Can you work these out from the model? Positions are in its coordinate system, mm. Face numbers are marked on the shaded views. A direction names the side the tool comes from. Give positions to 0.01 mm unless a question says otherwise; leave off trailing zeros. Write each loop counter-clockwise with the first axis right and the second up, starting at its lowest first coordinate (ties: lowest second). Pieces come first, ordered by that corner, then holes.
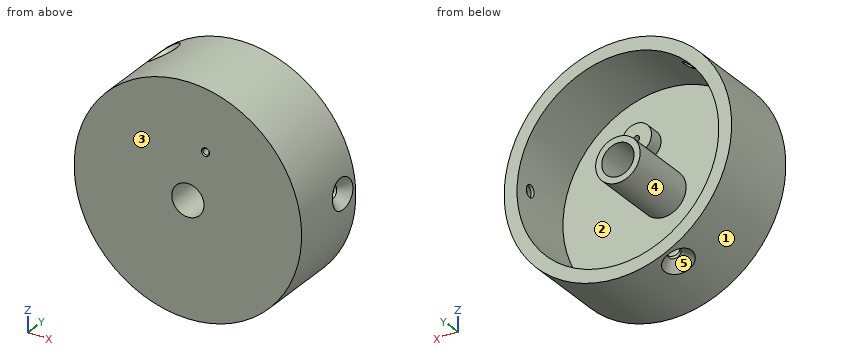
```python
from build123d import *

# Parameters (mm, degrees)
SKETCH1_R                     = 23
BOSS_EXTRUDE1_DEPTH           = 17
SHELL1_T                      = -2.6
SKETCH4_R                     = 4.5
BOSS_EXTRUDE3_DEPTH           = 14.4
SKETCH5_R                     = 3.265
CUT_EXTRUDE2_DEPTH            = 37.701498607
CIRPATTERN1_COUNT             = 3
SKETCH14_R                    = 3
BOSS_EXTRUDE7_DEPTH           = 3
M1_6_TAPPED_HOLE1_D           = 1.25
M1_6_TAPPED_HOLE1_CSINK_D     = 1.65
M1_6_TAPPED_HOLE1_CSINK_ANGLE = 90


with BuildPart() as part:
    # Sketch1 → Boss-Extrude1 (new body)
    with BuildSketch(Plane(origin=(0, 0, 0), x_dir=(1, 0, 0), z_dir=(0, 1, 0))):
        with Locations(Location((0, 0, 0), (0, 0, 270))):
            Circle(SKETCH1_R)
    extrude(amount=BOSS_EXTRUDE1_DEPTH)

    # Shell1
    shell1_openings = [part.faces().sort_by_distance(p)[0] for p in [
        (0, 17, 0),
    ]]
    offset(amount=SHELL1_T, openings=shell1_openings, kind=Kind.INTERSECTION)

    # Sketch4 → Boss-Extrude3 (add)
    with BuildSketch(Plane(origin=(0, 2.6, 0), x_dir=(1, 0, 0), z_dir=(0, 1, 0))):
        with Locations(Location((0, 0, 0), (0, 0, 90))):
            Circle(SKETCH4_R)
    extrude(amount=BOSS_EXTRUDE3_DEPTH)

    # Sketch5 → Cut-Extrude2 (cut, through all)
    with BuildSketch(Plane(origin=(0, 17, 0), x_dir=(1, 0, 0), z_dir=(0, 1, 0))):
        with Locations(Location((0, 0, 0), (0, 0, 270))):
            Circle(SKETCH5_R)
    extrude(amount=-CUT_EXTRUDE2_DEPTH, mode=Mode.SUBTRACT)

    # Sketch9 → CSK SLOT for M2 Countersunk Flat Head Screw1 (revolve, cut)
    with BuildSketch(Plane(origin=(22.911051483, 13, 2.020821599), x_dir=(0.08786180866791495, 0, -0.9961326731804369), z_dir=(0, 1, 0))):
        Polygon((0, 0), (0, 5.721032743), (1.2, 5), (1.2, 2), (3.2, 0), align=None)
    csk_slot_for_m2_countersunk_flat_head_sc = revolve(axis=Axis((29.236493958, 13, 2.578744084), (-0.9961326731804366, 0, -0.08786180866791493)), mode=Mode.SUBTRACT)

    # CirPattern1: CSK SLOT for M2 Countersunk Flat Head Screw1 ×3 about axis
    cirpattern1_axis = Axis((0, 17, 0), (0, -1, 0))
    for i in range(1, CIRPATTERN1_COUNT):
        add(csk_slot_for_m2_countersunk_flat_head_sc.rotate(cirpattern1_axis, i * 360 / CIRPATTERN1_COUNT), mode=Mode.SUBTRACT)

    # Sketch14 → Boss-Extrude7 (add)
    with BuildSketch(Plane(origin=(0, 2.6, 0), x_dir=(1, 0, 0), z_dir=(0, 1, 0))):
        with Locations(Location((3.564798354, -10.406354438, 0), (0, 0, 270))):
            Circle(SKETCH14_R)
    extrude(amount=BOSS_EXTRUDE7_DEPTH)

    # M1.6 Tapped Hole1 (through all)
    with Locations(Plane(origin=(0, 0, 0), x_dir=(-1, 0, 0), z_dir=(0, -1, 0))):
        with Locations((-3.564798354, -10.406354438)):
            CounterSinkHole(M1_6_TAPPED_HOLE1_D / 2, M1_6_TAPPED_HOLE1_CSINK_D / 2, counter_sink_angle=M1_6_TAPPED_HOLE1_CSINK_ANGLE)


solid = part.part
```
1) For the marked faces 4 and 5, which set-ups out of +Z, -Z, +X, -X, +Y, -Y let a thin tool reach every point of the face, with its end or its side?
Values follow:
face 4: +Y
face 5: -Z
2) Suppose I cut it at D-D on x = 17. Write out the boundary of the cut face in (y, z), plus the area to 3 significant figures.
Values follow:
outline: (0, -15.49) - (17, -15.49) - (17, -11.28) - (2.6, -11.28) - (2.6, 11.28) - (17, 11.28) - (17, 15.49) - (0, 15.49) - close
area: 202 mm2
3) For pin 1 Ø1.5 at (y, z) = (7.5, -8.5) entering from -X; pin 2 Ø3 at (x, y) = (16, 11) entering from -Z; pin 3 Ø4 at (x, y) = (-13.5, 11) entering from +Z, each with a flat end and sliding along its axis, tell me the tip position at first contact or that it passes through.
Values follow:
pin 1: stops at x = -21.65
pin 2: stops at z = -17.85
pin 3: stops at z = 19.89
4) Please list where these lines run through material, in increasing order: L1, parallel to X at y = 12.75, z = 0 (3 decimals); L2, parallel to X at y = 10.75, z = 0 (3 decimals); L3, parallel to Z at x = -1.5, y = 11.5.
Values follow:
L1: x = -23 to -20.4, -4.5 to -3.265, 3.265 to 4.5, 20.4 to 21.818
L2: x = -23 to -20.4, -4.5 to -3.265, 3.265 to 4.5, 20.4 to 22.907
L3: z = -22.95 to -20.34, -4.24 to -2.9, 2.9 to 4.24, 20.34 to 22.95
5) Suppose I cut it at B-B on y = 8.25. Write out the boundary of the cut face in (x, z) (3 decimals), plus the area to 3 significant figures.
Values follow:
outline: circle Ø46 at (0, 0); circle Ø9 at (0, 0); hole circle Ø40.8 at (0, 0); hole circle Ø6.53 at (0, 0)
area: 385 mm2
6) If we mould it in two halves opening along Z, with no side actions, what happens to the marked faces 1, 2 and 3? For each: +Z half, -Z half, draft (parallel to the pull), parting line (faces both ways), or undercut.
Values follow:
face 1: parting line
face 2: undercut
face 3: draft
7) Suppose I cut it at A-A on y = 5. Write out the boundary of the cut face in (x, z) (3 decimals).
Values follow:
outline: circle Ø46 at (0, 0); circle Ø9 at (0, 0); circle Ø6 at (3.565, 10.406); hole circle Ø40.8 at (0, 0); hole circle Ø6.53 at (0, 0); hole circle Ø1.25 at (3.565, 10.406)
8) Suppose I cut it at C-C on z = -2. Write out the boundary of the cut face in (x, y), plus the area to 3 significant figures.
Values follow:
outline: (-22.91, 0) - (-2.58, 0) - (-2.58, 17) - (-4.03, 17) - (-4.03, 2.6) - (-20.3, 2.6) - (-20.3, 17) - (-22.91, 17) - close; (2.58, 0) - (22.91, 0) - (22.91, 17) - (20.3, 17) - (20.3, 2.6) - (4.03, 2.6) - (4.03, 17) - (2.58, 17) - close
area: 223 mm2
